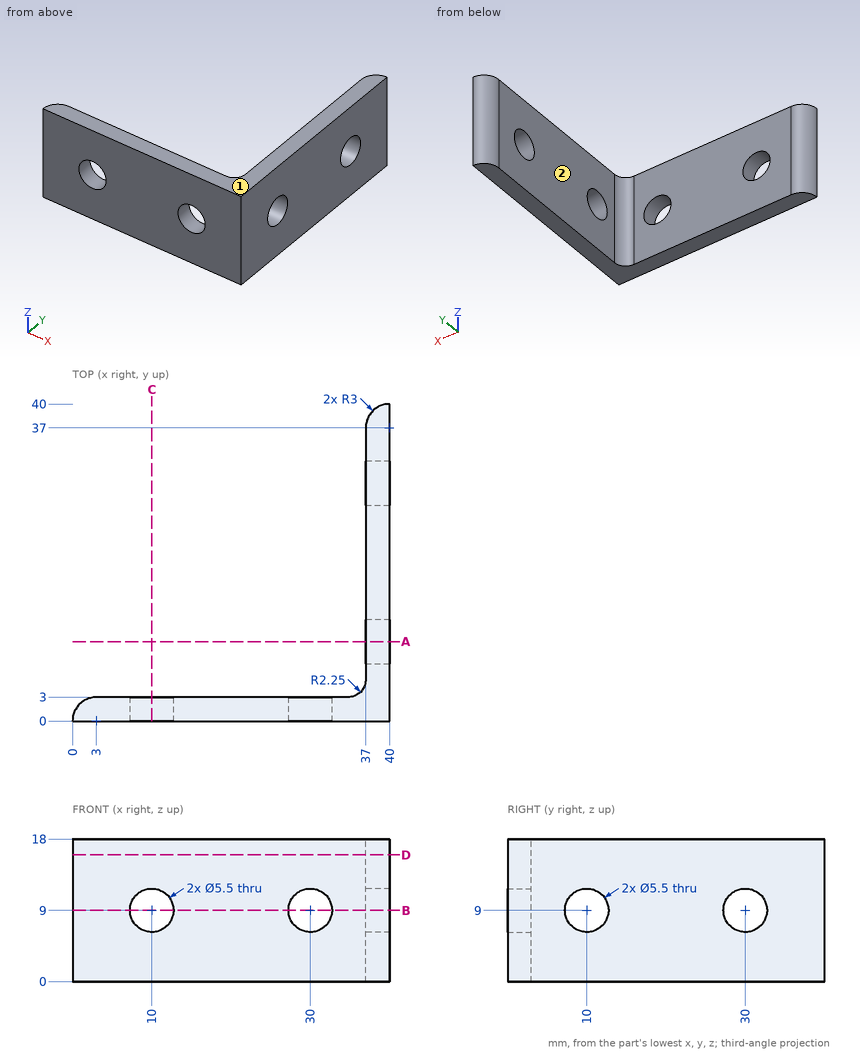
Drawing for the job (mm, zero at the part's lowest x, y, z). A direction names the side the tool comes from. Round coordinates to 2 decimals unless told otherwise and drop trailing zeros. Loops run counter-clockwise (first coordinate to the right, second up) from the corner with the lowest first, then second, coordinate; pieces in that order, holes last. Notation, with made-up numbers: M 17,75 L 63,75 A20 ccw 63,107 Z; hole C -28.75,58 d8. An arc over 180 degrees is marked long. Use a Markdown table: item, result. Add a question column.
(1) Which spindle directions (+Z, -Z, +X, -X, +Y, -Y) get a long thin tool onto all of the face, cutting with end or side? Do the marked faces 1 and 2. Say none if no direction does.
(2) Drill centre lines: line 1 (Z direction, x = 38, y = 30); line 2 (X direction, y = 21, z = 8.5); line 3 (Y direction, x = 12.5, z = 14.75). Where is each one in solid material? Low to high.
(3) Cut at C-C (x = 10). Give the cut face in (y, z).
(4) Cut at B-B (z = 9). Give the cut face in (x, y).
(5) Cut at D-D (z = 16). Give the cut face in (x, y), and give its area (3 significant figures).
(6) Flat gauge pins, fed straight in: pin 1 (1.5 mm diameter, centred on y = 7, z = 3.5, fed in from -X); pin 2 (7 mm diameter, centred on x = 30, z = 9, fed in from -Y); pin 3 (3 mm diameter, centred on x = 31, z = 10, fed in from +Y). Where does each tip first touch, or does it go through?
(7) Cut at A-A (y = 10). Give the cut face in (x, z).
Geometry says:
| question | item | result |
|---|---|---|
| 1 | face 1 | +Z, +X, -X, +Y, -Y |
| 1 | face 2 | +Z, -Z, -X, +Y |
| 2 | line 1 | z = 0 to 6.25, 11.75 to 18 |
| 2 | line 2 | x = 37 to 40 |
| 2 | line 3 | y = 0 to 3 |
| 3 | outline | M 0,0 L 3,0 L 3,6.25 L 0,6.25 Z; M 0,11.75 L 3,11.75 L 3,18 L 0,18 Z |
| 4 | outline | M 0,0 L 7.25,0 L 7.25,3 L 3,3 A3 ccw Z; M 12.75,0 L 27.25,0 L 27.25,3 L 12.75,3 Z; M 32.75,0 L 40,0 L 40,7.25 L 37,7.25 L 37,5.25 A2.25 cw 34.75,3 L 32.75,3 Z; M 37,12.75 L 40,12.75 L 40,27.25 L 37,27.25 Z; M 37,32.75 L 40,32.75 L 40,40 A3 ccw 37,37 Z |
| 5 | outline | M 0,0 L 40,0 L 40,40 A3 ccw 37,37 L 37,5.25 A2.25 cw 34.75,3 L 3,3 A3 ccw Z |
| 5 | area | 228 mm² |
| 6 | pin 1 | stops at x = 37 |
| 6 | pin 2 | stops at y = 0 |
| 6 | pin 3 | stops at y = 3 |
| 7 | outline | M 37,0 L 40,0 L 40,6.25 L 37,6.25 Z; M 37,11.75 L 40,11.75 L 40,18 L 37,18 Z |
